Answer from the drawing. Dimensions are ordinates in mm from the lowest x, y and z of the part. Coordinates: 2 decimals unless noted, no trailing zeros. Loops run counter-clockwise (first coordinate to the right, second up) from the corner with the lowest first, then second, coordinate; pieces in that order, holes last. Notation, with made-up numbers: (-6, 30.5) - (14, 30.5) arc R19 ccw to (14, 37.5) - close; hole circle Ø10 at (75.25, 19.5). An arc over 180 degrees is marked (long way). Use one line per item in the form item = value. Start each with the question number.
1) A cutting plane is placed at B-B (y = 43). Give the vertices of the cut face in (x, z), and give its area (3 significant figures).
2) A cutting plane is placed at A-A (x = 50). Give the vertices of the cut face in (y, z).
3) Each of these flat-tipped pins is pushed along its axis until it touches: P1, Ø4.5, axis at y = 36.5, z = 10.5, coming from the -X side; P2, Ø1.2, axis at x = 58.5, z = 11.5, coming from the -Y side; P3, Ø6.5, axis at x = 51.5, y = 43, coming from the +Z side; P4, Ø2, axis at x = 42, z = 10.5, coming from the -Y side. Where does it stop, or does it pass through?
4) The mould has two halves that part along X. Classify the marked faces 1, 2 and 3: released by +X, released by -X, zero draft, split by the parting line, or undercut.
5) Consider line 1 (X direction, y = 53.5, z = 12); line 2 (X direction, y = 27, z = 9); line 3 (Y direction, x = 19.5, z = 4.75). Determine where each line is inside the solid, lowest interval first.
6) A cutting plane is placed at C-C (z = 11.5). Give the vertices of the cut face in (x, y), and give its area (3 significant figures).
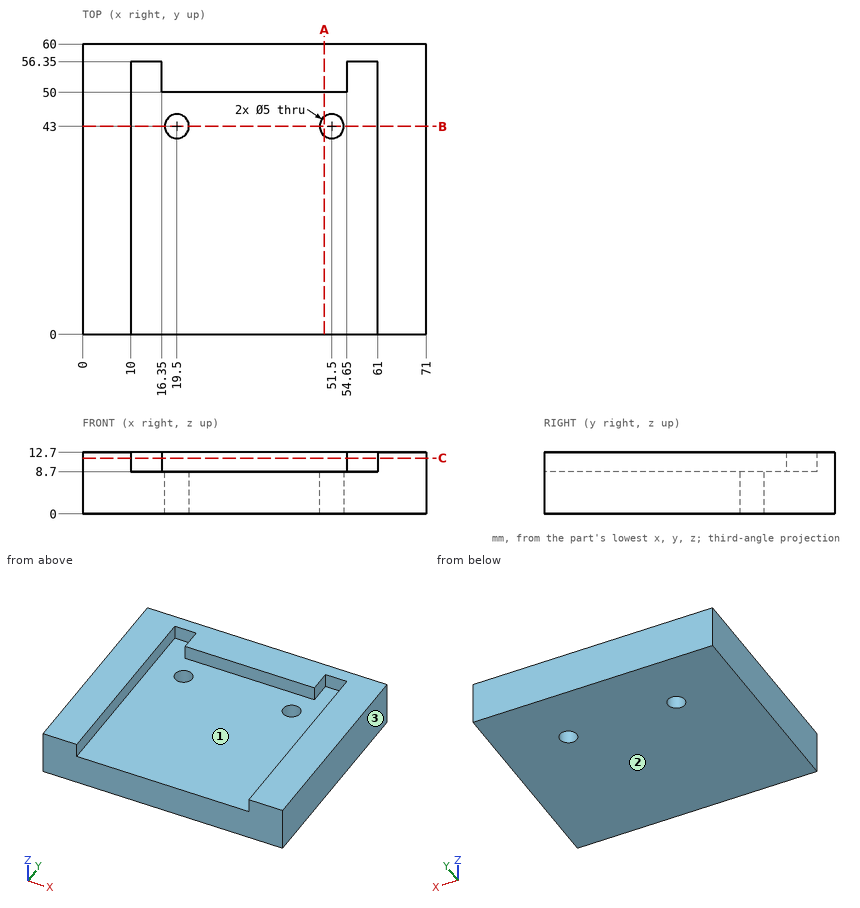
Found:
q1.outline = (0, 0) - (17, 0) - (17, 8.7) - (10, 8.7) - (10, 12.7) - (0, 12.7) - close; (22, 0) - (49, 0) - (49, 8.7) - (22, 8.7) - close; (54, 0) - (71, 0) - (71, 12.7) - (61, 12.7) - (61, 8.7) - (54, 8.7) - close
q1.area = 611 mm^2
q2.outline = (0, 0) - (41, 0) - (41, 8.7) - (0, 8.7) - close; (45, 0) - (60, 0) - (60, 12.7) - (50, 12.7) - (50, 8.7) - (45, 8.7) - close
q3.P1 = 0
q3.P2 = 56.35
q3.P3 = 8.7
q3.P4 = 50
q4.face_1 = undercut
q4.face_2 = zero draft
q4.face_3 = released by +X
q5.line_1 = 0 to 10, 16.35 to 54.65, 61 to 71
q5.line_2 = 0 to 10, 61 to 71
q5.line_3 = 0 to 40.5, 45.5 to 60
q6.outline = (0, 0) - (10, 0) - (10, 56.35) - (16.35, 56.35) - (16.35, 50) - (54.65, 50) - (54.65, 56.35) - (61, 56.35) - (61, 0) - (71, 0) - (71, 60) - (0, 60) - close
q6.area = 1,630 mm^2
